Could you check a few things on this model? Use its own coordinates, in mm. Give positions to 0.01 mm unless a question says otherwise; leave off trailing zeros. Loops run counter-clockwise (first coordinate to the right, second up) from the corner with the lowest first, then second, coordinate; pieces in that order, holes last. Notation, with made-up numbers: M -7.75,70.25 L 16.25,70.25 A24 ccw 16.25,81.25 Z; hole C 16,32 d10. An arc over 180 degrees is marked long. Write each question's results on one line, items separated by ' | '. Start each with the question number.
Solid Edge part; units mm, degrees
sketch "Sketch1" plane through (0, 0, 0) normal (0, 0, 1) x (1, 0, 0)
  line L0 (-60, -60) -> (60, -60)
  line L1 (60, -60) -> (60, 60)
  line L2 (60, 60) -> (-60, 60)
  line L3 (-60, 60) -> (-60, -60)
extrude "Extrusionsausprägung_20" add sketch "Sketch1" along normal blind 10
hole "Bohrung_4" at (34, -34, 10) direction (0, 0, -1) diameter 7 end up to next countersink diameter 13.71 countersink angle 90
hole "Hole1" at (34, 34, 10) direction (0, 0, -1) diameter 7 end up to next countersink diameter 13.71 countersink angle 90
hole "Hole2" at (-34, 34, 10) direction (0, 0, -1) diameter 7 end up to next countersink diameter 13.71 countersink angle 90
hole "Hole3" at (-34, -34, 10) direction (0, 0, -1) diameter 7 end up to next countersink diameter 13.71 countersink angle 90
hole "Bohrung_12" at (-50, -50, 0) direction (0, 0, 1) diameter 6.6 end up to next
hole "Hole4" at (50, -50, 0) direction (0, 0, 1) diameter 6.6 end up to next
hole "Hole5" at (50, 50, 0) direction (0, 0, 1) diameter 6.6 end up to next
hole "Hole6" at (-50, 50, 0) direction (0, 0, 1) diameter 6.6 end up to next
1) If we section it at D-D on y = 34: Write out the boundary of the cut face in (x, z) (3 decimals).
2) Thinking about a two-plate mould opening in Y: for faces 1 (the face through (60, -1, 5)), 2 (the face through (1, 60, 5)), 3 (the face through (-47.77, 47.57, 4.93)), 4 (the face through (37.47, 34.46, 3.37)), which applies, pulls with the +Y half, pulls with the -Y half, needs draft (parallel to the pull), parting line crosses it, or undercut?
3) I'm going to push flat-ended pins straight in: P1, Ø4, axis at x = 50, y = 50, coming from the -Z side; P2, Ø7.5, axis at x = -50, y = 50, coming from the +Z side. Where does each tip first touch, or does it pass through?
4) Please list where these lines run through material, in increasing order: line 1 (Y direction, x = 34, z = 3); line 2 (Y direction, x = -50, z = 7.75). Write a range as from..to.
5) If we section it at A-A on y = 50: Write out the boundary of the cut face in (x, z), plus the area to 3 significant figures.
6) If we section it at C-C on z = 3: State how many separate pieces and enclosed holes the cut face has, plus the area to 3 significant figures.
Calculated:
1) outline: M -60,0 L -37.5,0 L -37.5,6.645 L -40.855,10 L -60,10 Z; M -30.5,0 L 30.5,0 L 30.5,6.645 L 27.145,10 L -27.145,10 L -30.5,6.645 Z; M 37.5,0 L 60,0 L 60,10 L 40.855,10 L 37.5,6.645 Z
2) face 1: needs draft | face 2: pulls with the +Y half | face 3: undercut | face 4: undercut
3) P1: passes through | P2: stops at z = 10
4) line 1: y = -60..-37.5, -30.5..30.5, 37.5..60 | line 2: y = -60..-53.3, -46.7..46.7, 53.3..60
5) outline: M -60,0 L -53.3,0 L -53.3,10 L -60,10 Z; M -46.7,0 L 46.7,0 L 46.7,10 L -46.7,10 Z; M 53.3,0 L 60,0 L 60,10 L 53.3,10 Z | area: 1,070 mm2
6) separate pieces: 1 | enclosed holes: 8 | area: 14,100 mm2
